from build123d import *

# Parameters (mm, degrees)
SKETCH1_R               = 7.5
BOSS_EXTRUDE1_DEPTH     = 58
SKETCH2_W               = 17.33939444
SKETCH2_H               = 30
CUT_EXTRUDE1_DEPTH      = 107.60206377
CUT_EXTRUDE5_DEPTH      = 107.60206377
CUT_EXTRUDE5_DEPTH_BACK = 107.60206377
SKETCH3_R               = 7
CUT_EXTRUDE8_DEPTH      = 6
CUT_EXTRUDE9_DEPTH      = 12


with BuildPart() as part:
    # Sketch1 → Boss-Extrude1 (new body)
    with BuildSketch(Plane.XY):
        with BuildLine():
            Line((0, 0), (0, 24))
            ThreePointArc((0, 24), (16.66060556, 35.82575695), (36.66060556, 40))
            Line((36.66060556, 40), (65, 40))
            Line((65, 40), (80, 31.339745962))
            Line((80, 31.339745962), (80, 8.660254038))
            Line((80, 8.660254038), (65, 0))
            Line((65, 0), (0, 0))
        make_face()
        with Locations(Location((34, 19, 0), (0, 0, 180))):
            Circle(SKETCH1_R, mode=Mode.SUBTRACT)
    extrude(amount=BOSS_EXTRUDE1_DEPTH)

    # Sketch2 → Cut-Extrude1 (cut, through all)
    with BuildSketch(Plane(origin=(0, 40, 0), x_dir=(1, 0, 0), z_dir=(0, 1, 0))):
        Polygon((16, -8), (0, -8), (0, -50), (16, -50), (16, -44), (36.66060556, -44), (36.66060556, -14), (16, -14), align=None)
        with Locations((45.33030278, -29)):
            Rectangle(SKETCH2_W, SKETCH2_H)
        Polygon((80, 0), (65, 0), (80, -15), align=None)
        Polygon((80, -58), (80, -43), (65, -58), align=None)
    extrude(amount=-CUT_EXTRUDE1_DEPTH, mode=Mode.SUBTRACT)

    # Sketch3 → Cut-Extrude5 (cut, two sides: drawn at the far end of the back side and taken through both)
    with BuildSketch(Plane(origin=(80, 0, 0), x_dir=(0, 0, -1), z_dir=(1, 0, 0)).offset(-CUT_EXTRUDE5_DEPTH_BACK)):
        with Locations(Location((-29, 20, 0), (0, 0, 270))):
            Circle(SKETCH3_R)
    extrude(amount=CUT_EXTRUDE5_DEPTH + CUT_EXTRUDE5_DEPTH_BACK, mode=Mode.SUBTRACT)

    # Sketch7 → Cut-Extrude8 (cut)
    with BuildSketch(Plane.XY.offset(58)):
        with BuildLine():
            Line((16.452013389, 2), (16.452013389, 33.538635744))
            ThreePointArc((16.452013389, 33.538635744), (8.428320966, 28.819300697), (1.466424222, 22.64))
            ThreePointArc((1.466424222, 22.64), (0.7236706, 21.820381922), (0, 20.98386677))
            Line((0, 20.98386677), (0, 2))
            Line((0, 2), (16.452013389, 2))
        make_face()
    cut_extrude8 = extrude(amount=-CUT_EXTRUDE8_DEPTH, mode=Mode.SUBTRACT)

    # Sketch7<3> → Cut-Extrude9 (cut)
    with BuildSketch(Plane.XY.offset(58)):
        with BuildLine():
            ThreePointArc((36.66060556, 38), (26.3130096, 36.871390612), (16.452013389, 33.538635744))
            Line((16.452013389, 33.538635744), (16.452013389, 2))
            Line((16.452013389, 2), (63, 2))
            Line((63, 2), (63, 38))
            Line((63, 38), (36.66060556, 38))
        make_face()
    cut_extrude9 = extrude(amount=-CUT_EXTRUDE9_DEPTH, mode=Mode.SUBTRACT)

    # Mirror3: Cut-Extrude8, Cut-Extrude9 across plane
    add(cut_extrude8.mirror(Plane.XY.offset(29)), mode=Mode.SUBTRACT)
    add(cut_extrude9.mirror(Plane.XY.offset(29)), mode=Mode.SUBTRACT)


solid = part.part
Geometry check sheet. Reference: the model listing, model coordinates, mm. A direction names the side the tool comes from. Give positions to 0.01 mm unless a question says otherwise; leave off trailing zeros. Order: outer loops, then holes, each group sorted by start corner. A loop starts at its lowest first (then second) coordinate and runs counter-clockwise, first axis right, second up. Notation, with made-up numbers: (-34.75, 38) - (-25.75, 38) arc R19 ccw to (-25.75, 71) - close; hole circle Ø8 at (0, -24.5). An arc over 180 degrees is marked (long way). Use one line per item in the form item = value.
1) Sectioned sample at A-A (x = 55). Record the boundary of the cut face in (y, z).
Working result:
outline = (0, 0) - (2, 0) - (2, 12) - (38, 12) - (38, 0) - (40, 0) - (40, 58) - (38, 58) - (38, 46) - (2, 46) - (2, 58) - (0, 58) - close; hole circle Ø14 at (20, 29)
2) Depth check by flat-ended pin: pin 1 Ø13 at (x, z) = (56, 4) entering from -Y; pin 2 Ø5 at (x, y) = (4, 21) entering from -Z; pin 3 Ø1.8 at (y, z) = (15, 48) entering from -X; pin 4 Ø5 at (y, z) = (15, 9.5) entering from +X. Enter the tip coordinate at first touch or a pass-through.
Working result:
pin_1 = 0
pin_2 = 6
pin_3 = 16
pin_4 = 77
3) Draft check along Z on faces 1 (the face through (57, 40, 29)), 2 (the face through (45, 20, 12)), 3 (the face through (66.818, 21.517, 35.834)). Enter one of: released by +Z, released by -Z, zero draft, split by the parting line, or undercut.
Working result:
face_1 = zero draft
face_2 = released by -Z
face_3 = undercut
4) Sectioned sample at B-B (z = 29). Record the boundary of the cut face in (x, y).
Working result:
outline = (54, 0) - (65, 0) - (80, 8.66) - (80, 13) - (54, 13) - close; (54, 27) - (80, 27) - (80, 31.34) - (65, 40) - (54, 40) - close
5) Material ranges on probe 1 along Y at (x, z) = (36.5, 5.5); probe 2 along Z at (x, y) = (16.5, 12.5); probe 3 along Z at (x, y) = (13, 22), recorded low to high. Write a range as from..to.
Working result:
probe_1 = 0..2, 38..40
probe_2 = 12..14, 44..46
probe_3 = 6..8, 50..52
6) Sectioned sample at C-C (y = 19). Count the separate pieces of the cut face and the enclosed holes in it, and give its area (3 significant figures).
Working result:
separate_pieces = 4
enclosed_holes = 0
area = 868 mm^2
7) Sectioned sample at D-D (x = 15). Record the boundary of the cut face in (y, z).
Working result:
outline = (0, 0) - (2, 0) - (2, 6) - (32.83, 6) - (32.83, 0) - (35.06, 0) - (35.06, 8) - (0, 8) - close; (0, 50) - (35.06, 50) - (35.06, 58) - (32.83, 58) - (32.83, 52) - (2, 52) - (2, 58) - (0, 58) - close
8) Access from +Z, -Z, +X, -X, +Y, -Y to the whole of each face (thin tool, end or side, straight path). Record for faces 4 (the face through (16.452, 18, 9)), 5 (the face through (39, 25, 14)), 6 (the face through (0, 12, 51)), 7 (the face through (50, 38, 52)).
Working result:
face_4 = -Z
face_5 = -X, +Y, -Y
face_6 = +Z, -Z, -X, +Y, -Y
face_7 = +Z
